from build123d import *


with BuildPart() as f1:
    # F0 (on Right) → F1 (revolve)
    with BuildSketch(Plane.YZ):
        Polygon((0, 3.0734), (0, 0), (25.4, 0), (46.337384, 41.874768), (47.039628, 43.279255), (47.778658, 44.757316), (48.688656, 46.577311), (50.8, 50.8), (47.363834, 50.8), (23.500534, 3.0734), align=None)
        Polygon((47.039628, 43.279255), (46.337384, 41.874768), (47.039628, 41.874768), align=None)
        Polygon((47.778658, 44.757316), (47.039628, 43.279255), (47.778658, 43.279255), align=None)
        Polygon((48.688656, 46.577311), (47.778658, 44.757316), (48.688656, 44.757316), align=None)
    revolve(axis=Axis((0, 0, 25.4), (0, 0, 1)))


solid = f1.part
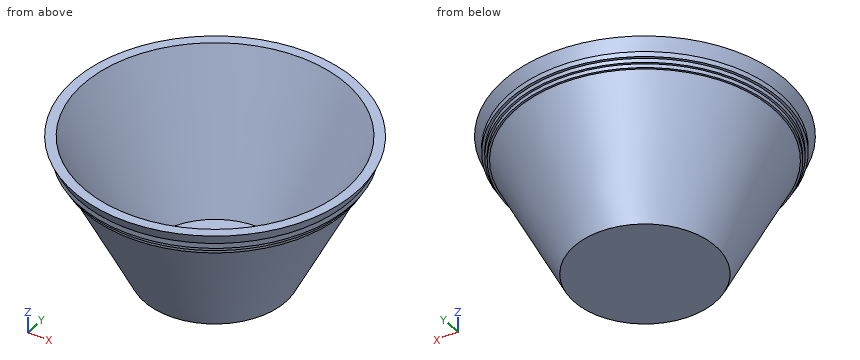
Geometry check sheet. Reference: the model listing, model coordinates, mm. Coordinates: 2 decimals unless noted, no trailing zeros. Order: outer loops, then holes, each group sorted by start corner. A loop starts at its lowest first (then second) coordinate and runs counter-clockwise, first axis right, second up. Notation, with made-up numbers: (3, -20) - (29, -20) arc R21 cw to (29, -6) - close; hole circle Ø1 at (87.25, -29). An arc over 180 degrees is marked (long way). Answer in a Markdown table with one row per item. Add a question column.
1) Cross-section at C-C, the plane z = 33.5. Record the cut outline in (x, y), then the cut area to 3 significant figures.
2) Cross-section at D-D, the plane z = 19. Record the cut outline in (x, y), then the cut area to 3 significant figures.
3) Gauge pin test, flat ends, axial feed: P1, Ø1, axis at x = 33.5, y = 26, coming from the +Z side; P2, Ø10, axis at y = -34, z = 19, coming from the -X side; P3, Ø10, axis at y = -23, z = 7.5, coming from the +X side. Record the tip position at first contact, or that the pin passes through.
4) Cross-section at A-A, the plane x = 0. Record the cut outline in (y, z), then the cut area to 3 significant figures.
5) Material ranges on line 1 along X through (y, z) = (5, 19); line 2 along Y through (x, z) = (-34, 46.5); line 3 along Y through (x, z) = (-35, 34.5), recorded low to high. Write a range as [from, to].
Check result:
| question | item | result |
|---|---|---|
| 1 | outline | circle Ø84.3 at (0, 0); hole circle Ø77.43 at (0, 0) |
| 1 | area | 873 mm² |
| 2 | outline | circle Ø69.8 at (0, 0); hole circle Ø62.93 at (0, 0) |
| 2 | area | 716 mm² |
| 3 | P1 | stops at z = 41.88 |
| 3 | P2 | stops at x = -20.65 |
| 3 | P3 | stops at x = 24.05 |
| 4 | outline | (-50.8, 50.8) - (-48.69, 46.58) - (-48.69, 44.76) - (-47.78, 44.76) - (-47.78, 43.28) - (-47.04, 43.28) - (-47.04, 41.87) - (-46.34, 41.87) - (-25.4, 0) - (25.4, 0) - (46.34, 41.87) - (47.04, 41.87) - (47.04, 43.28) - (47.78, 43.28) - (47.78, 44.76) - (48.69, 44.76) - (48.69, 46.58) - (50.8, 50.8) - (47.36, 50.8) - (23.5, 3.07) - (-23.5, 3.07) - (-47.36, 50.8) - close |
| 4 | area | 493 mm² |
| 5 | line 1 | x = [-34.54, -31.06], [31.06, 34.54] |
| 5 | line 2 | y = [-34.85, -29.8], [29.8, 34.85] |
| 5 | line 3 | y = [-24.37, -17.68], [17.68, 24.37] |
